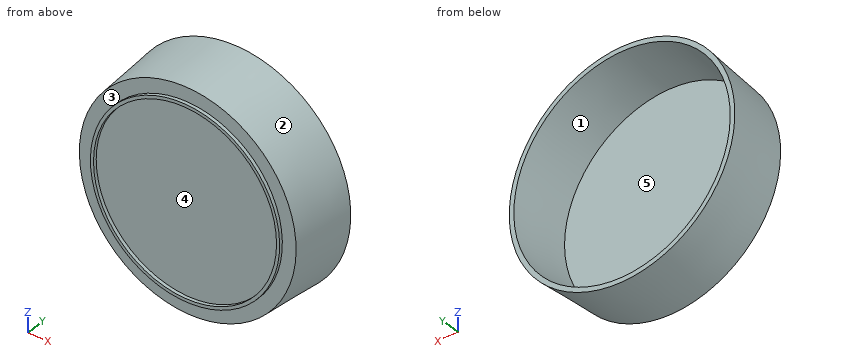
```python
from build123d import *

# Parameters (mm, degrees)
SHELL1_T            = -1.016
SKETCH3_R           = 20.9741
SKETCH3_R_2         = 20.2883
BOSS_EXTRUDE1_DEPTH = 0.762


with BuildPart() as part:
    # Sketch2 → Revolve1 (revolve)
    with BuildSketch(Plane.XY, mode=Mode.PRIVATE) as revolve1_sk:
        Polygon((0, 0), (24.0221, 0), (25, 14.1224), (0, 14.1224), align=None)
    revolve(revolve1_sk.sketch.rotate(Axis((0, 0, 0), (0, 1, 0)), 90), axis=Axis((0, 0, 0), (0, 1, 0)))

    # Shell1
    shell1_openings = [part.faces().sort_by_distance(p)[0] for p in [
        (0, 14.1224, 0),
    ]]
    offset(amount=SHELL1_T, openings=shell1_openings, kind=Kind.INTERSECTION)

    # Sketch3 → Boss-Extrude1 (add)
    with BuildSketch(Plane.XZ):
        with Locations(Location((0, 0, 0), (0, 0, 90))):
            Circle(SKETCH3_R)
        with Locations(Location((0, 0, 0), (0, 0, 90))):
            Circle(SKETCH3_R_2, mode=Mode.SUBTRACT)
    extrude(amount=BOSS_EXTRUDE1_DEPTH)


solid = part.part
```
Geometry: final body of the model. Coordinates: model frame, mm. Face numbers are marked on the shaded views. A direction names the side the tool comes from. Round coordinates to 2 decimals unless told otherwise and drop trailing zeros. Order: outer loops, then holes, each group sorted by start corner. A loop starts at its lowest first (then second) coordinate and runs counter-clockwise, first axis right, second up. Notation, with made-up numbers: (80.25, -38.75) -> (112.25, -38.75) arc R29 ccw to (112.25, -10.75) -> close; hole circle Ø9 at (68.25, 77). An arc over 180 degrees is marked (long way). Use one line per item in the form item = value.
(1) Draft query along X for the marked faces 1, 2 and 3. Return one class per face: pulls with the +X half, pulls with the -X half, needs draft (parallel to the pull), parting line crosses it, or undercut.
Results list:
face_1 = undercut
face_2 = parting line crosses it
face_3 = needs draft
(2) Section B-B on z = 0. Return loops of the section in (x, y).
Results list:
outline = (-25, 14.12) -> (-24.02, 0) -> (-20.97, 0) -> (-20.97, -0.76) -> (-20.29, -0.76) -> (-20.29, 0) -> (20.29, 0) -> (20.29, -0.76) -> (20.97, -0.76) -> (20.97, 0) -> (24.02, 0) -> (25, 14.12) -> (23.98, 14.12) -> (23.07, 1.02) -> (-23.07, 1.02) -> (-23.98, 14.12) -> close
(3) Ray query, probe 1 along X at (y, z) = (-0.3, 0); probe 2 along Y at (x, z) = (-15, 6.5); probe 3 along Z at (x, y) = (-9.5, 10.25). Return the intervals inside material, ascending. Write a range as [from, to].
Results list:
probe_1 = [-20.97, -20.29], [20.29, 20.97]
probe_2 = [0, 1.02]
probe_3 = [-22.83, -21.73], [21.73, 22.83]
(4) Section D-D on y = 7. Return loops of the section in (x, z), and give its area (3 significant figures).
Results list:
outline = circle Ø49.01 at (0, 0); hole circle Ø46.98 at (0, 0)
area = 154 mm^2
(5) First-contact query: pin 1 Ø2 at (x, z) = (-3, -3.5) entering from -Y; pin 2 Ø3 at (x, y) = (-8, 2) entering from +Z; pin 3 Ø8 at (y, z) = (7, 9.5) entering from -X. Flat tips, straight axial feed; report the tip coordinate or a pass-through.
Results list:
pin_1 = 0
pin_2 = 23.28
pin_3 = -23.92
(6) Section C-C on y = 13. Return loops of the section in (x, z), and give its area (3 significant figures).
Results list:
outline = circle Ø49.84 at (0, 0); hole circle Ø47.81 at (0, 0)
area = 156 mm^2
(7) Section A-A on x = 0. Return loops of the section in (y, z).
Results list:
outline = (-0.76, -20.97) -> (0, -20.97) -> (0, -24.02) -> (14.12, -25) -> (14.12, -23.98) -> (1.02, -23.07) -> (1.02, 23.07) -> (14.12, 23.98) -> (14.12, 25) -> (0, 24.02) -> (0, 20.97) -> (-0.76, 20.97) -> (-0.76, 20.29) -> (0, 20.29) -> (0, -20.29) -> (-0.76, -20.29) -> close
(8) Access query for the marked faces 4 and 5. Directions: +Z, -Z, +X, -X, +Y, -Y. A direction counts if a zero-diameter tool reaches every point of the face in a straight line with its end or side. Return the directions, or none.
Results list:
face_4 = -Y
face_5 = +Y
